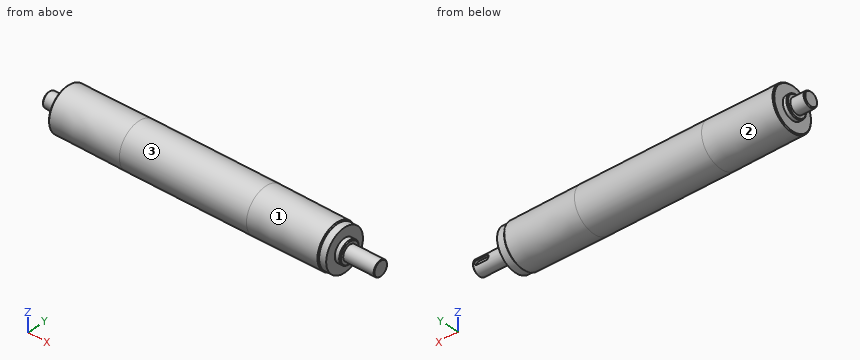
```python
from build123d import *

# Parameters (mm, degrees)
EXTRUDE1_DEPTH = 150


with BuildPart() as part:
    # Sketch1 → Revolve1 (revolve)
    with BuildSketch(Plane(origin=(0, 0, 0), x_dir=(1, 0, 0), z_dir=(0, 1, 0)), mode=Mode.PRIVATE) as revolve1_sk:
        Polygon((-72, 25), (72, 25), (152, 24.5), (153, 23.5), (161, 23.5), (161, 12.5), (166, 12.5), (167, 11.5), (167, 8.5), (201.5, 8.5), (202, 8), (202, 0), (-174, 0), (-174, 7.5), (-173, 8.5), (-158, 8.5), (-158, 11.5), (-157, 12.5), (-153, 12.5), (-153, 23.5), (-152, 24.5), align=None)
    revolve(revolve1_sk.sketch.rotate(Axis((-174, 0, 0), (1, 0, 0)), 180), axis=Axis((-174, 0, 0), (1, 0, 0)))  # turned: the seam where the file's is

    # Sketch2 → Extrude1 (cut)
    with BuildSketch(Plane(origin=(0, 5.5, 0), x_dir=(-1, 0, 0), z_dir=(0, 1, 0))):
        with BuildLine():
            Line((-197.5, 2.5), (-186.5, 2.5))
            ThreePointArc((-186.5, 2.5), (-184, 0), (-186.5, -2.5))
            Line((-186.5, -2.5), (-197.5, -2.5))
            ThreePointArc((-197.5, -2.5), (-200, 0), (-197.5, 2.5))
        make_face()
    extrude(amount=EXTRUDE1_DEPTH, mode=Mode.SUBTRACT)


solid = part.part
```
Build history of the part. All positions in model axes, mm. Face numbers are marked on the shaded views. A direction names the side the tool comes from. Round coordinates to 2 decimals unless told otherwise and drop trailing zeros. Loops run counter-clockwise (first coordinate to the right, second up) from the corner with the lowest first, then second, coordinate; pieces in that order, holes last.
Item 1: Saw through at B-B (x = -100). List the corners of the cut face in (y, z) (3 decimals), then the cut area to 3 significant figures.
Item 2: Which spindle directions (+Z, -Z, +X, -X, +Y, -Y) get a long thin tool onto all of the face, cutting with end or side? Do the marked faces 1, 2 and 3. Say none if no direction does.
Item 3: Saw through at A-A (x = -5). List the corners of the cut face in (y, z).
Item 4: Drill centre lines: line 1 along Y through (x, z) = (51, -5); line 2 along X through (y, z) = (-10, -17.5); line 3 along X through (y, z) = (-11, 1.5). Where is each one in solid material? Low to high.
Item 5: Pin check, flat tips, straight feed: P1, Ø12, axis at x = -105.5, z = -12.5, coming from the +Y side; P2, Ø1.5, axis at y = -6.5, z = -6.5, coming from the +X side; P3, Ø3, axis at x = 84.5, z = 11, coming from the +Y side. Stop position of each tip, or through.
Worked answers:
1. outline: circle Ø49.65 at (0, 0)
1. area: 1,940 mm2
2. face 1: +X
2. face 2: -X
2. face 3: +X, -X
3. outline: circle Ø50 at (0, 0)
4. line 1: y = -24.49 to 24.49
4. line 2: x = -153 to 161
4. line 3: x = -158 to 167
5. P1: stops at y = 23.92
5. P2: stops at x = 201.56
5. P3: stops at y = 23.04
